The model under review builds one solid part; all positions refer to its coordinate system, in mm. Round coordinates to 2 decimals unless told otherwise and drop trailing zeros. Order: outer loops, then holes, each group sorted by start corner. A loop starts at its lowest first (then second) coordinate and runs counter-clockwise, first axis right, second up.
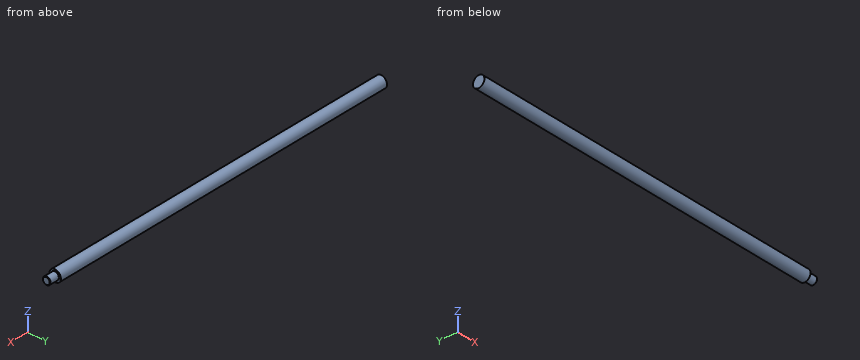
```python
from build123d import *


with BuildPart() as part:
    # Sketch1 → Revolve1 (revolve)
    with BuildSketch(Plane.XY):
        with BuildLine():
            Line((0, 6), (0, 0))
            Line((0, 0), (380, 0))
            Line((380, 0), (380, 3.5))
            Line((380, 3.5), (379.5, 4))
            Line((379.5, 4), (370.3, 4))
            ThreePointArc((370.3, 4), (370.087867966, 4.087867966), (370, 4.3))
            Line((370, 4.3), (370, 6))
            Line((370, 6), (0, 6))
        make_face()
    revolve(axis=Axis((0, 0, 0), (1, 0, 0)))


solid = part.part
```
(1) Insertion check: pin 1 (2 mm diameter, centred on x = 159, z = 2.5, fed in from -Y); pin 2 (3 mm diameter, centred on x = 260, z = 4, fed in from -Y); pin 3 (1 mm diameter, centred on x = 239, y = 2.5, fed in from +Z). Each pin has a flat end and moves straight along its axis. Give the tip position at first contact, or say it passes through.
Data:
pin 1: stops at y = -5.81
pin 2: stops at y = -5.45
pin 3: stops at z = 5.66
(2) Consider section A-A (x = 152). Write out the cut boundary in (y, z).
Data:
outline: circle Ø12 at (0, 0)
(3) To check wall thickness, follow probe 1 along X at (y, z) = (-4, 3); probe 2 along Y at (x, z) = (244.5, -4.25); probe 3 along Z at (x, y) = (30, 4.5). State the ranges of each line that lie inside material, in increasing order.
Data:
probe 1: x = 0 to 370
probe 2: y = -4.24 to 4.24
probe 3: z = -3.97 to 3.97
